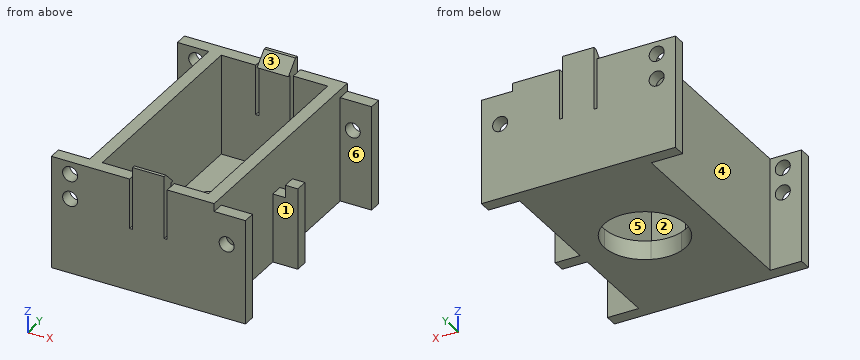
```python
from build123d import *

# Parameters (mm, degrees)
F1_DEPTH  = 2
F2_DEPTH  = 18
F3_DEPTH  = 3
F4_W      = 2
F4_H      = 5
F4_H_2    = 13
F5_DEPTH  = 5
F6_W      = 2
F6_H      = 16.7173967883
F7_DEPTH  = 5
F8_R      = 1.2
F9_DEPTH  = 40
F12_DEPTH = 1
F13_W     = 5
F13_H     = 2
F13_H_2   = 0.5
F14_DEPTH = 2
F15_SIZE  = 1.99999
F13_W_2   = 0.5
F16_DEPTH = 8


# Not quite as in the source:
# - a fillet or chamfer is up to 0.001 mm smaller than in the source, because OpenCascade refuses the exact size


with BuildPart() as f1:
    # F0 (on Top) → F1 (new body)
    with BuildSketch(Plane.XY):
        Polygon((-5.1606558692, 9.7513413054), (-11.6606558692, 9.7513413054), (-11.6606558692, -27.7486586946), (-5.1606558692, -27.7486586946), (2.8393441308, -27.7486586946), (9.3393441308, -27.7486586946), (9.3393441308, 9.7513413054), (2.8393441308, 9.7513413054), align=None)
        Polygon((-9.6606558692, -1.2486586946), (-9.6606558692, 7.7513413054), (7.3393441308, 7.7513413054), (7.3393441308, -1.2486586946), (7.3393441308, -16.7486586946), (7.3393441308, -25.7486586946), (-9.6606558692, -25.7486586946), (-9.6606558692, -16.7486586946), align=None, mode=Mode.SUBTRACT)
        with BuildLine():
            Line((3.3125979801, -16.7486586946), (-5.6339097184, -16.7486586946))
            ThreePointArc((-5.6339097184, -16.7486586946), (-2.8409986659, -25.1856853401), (4.3393441308, -19.9486586946))
            ThreePointArc((4.3393441308, -19.9486586946), (4.0763707763, -18.2683158979), (3.3125979801, -16.7486586946))
        make_face()
        with BuildLine():
            ThreePointArc((4.3393441308, 1.9513413054), (-2.8409986659, 7.1883679509), (-5.6339097184, -1.2486586946))
            Line((-5.6339097184, -1.2486586946), (3.3125979801, -1.2486586946))
            ThreePointArc((3.3125979801, -1.2486586946), (4.0763707763, 0.2709985087), (4.3393441308, 1.9513413054))
        make_face()
        with BuildLine():
            Line((7.3393441308, 7.7513413054), (-9.6606558692, 7.7513413054))
            Line((-9.6606558692, 7.7513413054), (-9.6606558692, -1.2486586946))
            Line((-9.6606558692, -1.2486586946), (-5.6339097184, -1.2486586946))
            ThreePointArc((-5.6339097184, -1.2486586946), (-2.8409986659, 7.1883679509), (4.3393441308, 1.9513413054))
            ThreePointArc((4.3393441308, 1.9513413054), (4.0763707763, 0.2709985087), (3.3125979801, -1.2486586946))
            Line((3.3125979801, -1.2486586946), (7.3393441308, -1.2486586946))
            Line((7.3393441308, -1.2486586946), (7.3393441308, 7.7513413054))
        make_face()
        with BuildLine():
            Line((-5.6339097184, -16.7486586946), (-9.6606558692, -16.7486586946))
            Line((-9.6606558692, -16.7486586946), (-9.6606558692, -25.7486586946))
            Line((-9.6606558692, -25.7486586946), (7.3393441308, -25.7486586946))
            Line((7.3393441308, -25.7486586946), (7.3393441308, -16.7486586946))
            Line((7.3393441308, -16.7486586946), (3.3125979801, -16.7486586946))
            ThreePointArc((3.3125979801, -16.7486586946), (4.0763707763, -18.2683158979), (4.3393441308, -19.9486586946))
            ThreePointArc((4.3393441308, -19.9486586946), (-2.8409986659, -25.1856853401), (-5.6339097184, -16.7486586946))
        make_face()
        with BuildLine():
            Line((7.3393441308, -16.7486586946), (7.3393441308, -1.2486586946))
            Line((7.3393441308, -1.2486586946), (3.3125979801, -1.2486586946))
            ThreePointArc((3.3125979801, -1.2486586946), (2.6358545698, -2.028169781), (1.8253711817, -2.667494311))
            ThreePointArc((1.8253711817, -2.667494311), (4.751289215, -5.2504717566), (5.8393441308, -8.9986586946))
            ThreePointArc((5.8393441308, -8.9986586946), (4.751289215, -12.7468456326), (1.8253711817, -15.3298230782))
            ThreePointArc((1.8253711817, -15.3298230782), (2.6358545698, -15.9691476082), (3.3125979801, -16.7486586946))
            Line((3.3125979801, -16.7486586946), (7.3393441308, -16.7486586946))
        make_face()
        with BuildLine():
            Line((-5.6339097184, -1.2486586946), (-9.6606558692, -1.2486586946))
            Line((-9.6606558692, -1.2486586946), (-9.6606558692, -16.7486586946))
            Line((-9.6606558692, -16.7486586946), (-5.6339097184, -16.7486586946))
            ThreePointArc((-5.6339097184, -16.7486586946), (-4.9571663082, -15.9691476082), (-4.14668292, -15.3298230782))
            ThreePointArc((-4.14668292, -15.3298230782), (-8.1606558692, -8.9986586946), (-4.14668292, -2.667494311))
            ThreePointArc((-4.14668292, -2.667494311), (-4.9571663082, -2.028169781), (-5.6339097184, -1.2486586946))
        make_face()
        with BuildLine():
            Line((3.3125979801, -1.2486586946), (-5.6339097184, -1.2486586946))
            ThreePointArc((-5.6339097184, -1.2486586946), (-4.9571663082, -2.028169781), (-4.14668292, -2.667494311))
            ThreePointArc((-4.14668292, -2.667494311), (-1.1606558692, -1.9986586946), (1.8253711817, -2.667494311))
            ThreePointArc((1.8253711817, -2.667494311), (2.6358545698, -2.028169781), (3.3125979801, -1.2486586946))
        make_face()
        with BuildLine():
            ThreePointArc((-4.14668292, -15.3298230782), (-4.9571663082, -15.9691476082), (-5.6339097184, -16.7486586946))
            Line((-5.6339097184, -16.7486586946), (3.3125979801, -16.7486586946))
            ThreePointArc((3.3125979801, -16.7486586946), (2.6358545698, -15.9691476082), (1.8253711817, -15.3298230782))
            ThreePointArc((1.8253711817, -15.3298230782), (-1.1606558692, -15.9986586946), (-4.14668292, -15.3298230782))
        make_face()
    extrude(amount=F1_DEPTH)

    # F0 (on Top) → F2 (join)
    with BuildSketch(Plane.XY):
        Polygon((-5.1606558692, 9.7513413054), (-11.6606558692, 9.7513413054), (-11.6606558692, -27.7486586946), (-5.1606558692, -27.7486586946), (2.8393441308, -27.7486586946), (9.3393441308, -27.7486586946), (9.3393441308, 9.7513413054), (2.8393441308, 9.7513413054), align=None)
        Polygon((-9.6606558692, -1.2486586946), (-9.6606558692, 7.7513413054), (7.3393441308, 7.7513413054), (7.3393441308, -1.2486586946), (7.3393441308, -16.7486586946), (7.3393441308, -25.7486586946), (-9.6606558692, -25.7486586946), (-9.6606558692, -16.7486586946), align=None, mode=Mode.SUBTRACT)
    extrude(amount=F2_DEPTH)

    # F0 (on Top) → F3 (join)
    with BuildSketch(Plane.XY):
        with BuildLine():
            ThreePointArc((-3.604859431, -2.9757134891), (-3.8801412786, -2.8292861752), (-4.14668292, -2.667494311))
            ThreePointArc((-4.14668292, -2.667494311), (-8.1606558692, -8.9986586946), (-4.14668292, -15.3298230782))
            ThreePointArc((-4.14668292, -15.3298230782), (-3.8801412786, -15.1680312141), (-3.604859431, -15.0216039001))
            ThreePointArc((-3.604859431, -15.0216039001), (-7.6606558692, -8.9986586946), (-3.604859431, -2.9757134891))
        make_face()
        with BuildLine():
            ThreePointArc((1.8253711817, -2.667494311), (-1.1606558692, -1.9986586946), (-4.14668292, -2.667494311))
            ThreePointArc((-4.14668292, -2.667494311), (-3.8801412786, -2.8292861752), (-3.604859431, -2.9757134891))
            ThreePointArc((-3.604859431, -2.9757134891), (-1.1606558692, -2.4986586946), (1.2835476927, -2.9757134891))
            ThreePointArc((1.2835476927, -2.9757134891), (1.5588295403, -2.8292861752), (1.8253711817, -2.667494311))
        make_face()
        with BuildLine():
            ThreePointArc((5.8393441308, -8.9986586946), (4.751289215, -5.2504717566), (1.8253711817, -2.667494311))
            ThreePointArc((1.8253711817, -2.667494311), (1.5588295403, -2.8292861752), (1.2835476927, -2.9757134891))
            ThreePointArc((1.2835476927, -2.9757134891), (4.2308802362, -5.3680473929), (5.3393441308, -8.9986586946))
            ThreePointArc((5.3393441308, -8.9986586946), (4.2308802362, -12.6292699963), (1.2835476927, -15.0216039001))
            ThreePointArc((1.2835476927, -15.0216039001), (1.5588295403, -15.1680312141), (1.8253711817, -15.3298230782))
            ThreePointArc((1.8253711817, -15.3298230782), (4.751289215, -12.7468456326), (5.8393441308, -8.9986586946))
        make_face()
        with BuildLine():
            ThreePointArc((-3.604859431, -15.0216039001), (-3.8801412786, -15.1680312141), (-4.14668292, -15.3298230782))
            ThreePointArc((-4.14668292, -15.3298230782), (-1.1606558692, -15.9986586946), (1.8253711817, -15.3298230782))
            ThreePointArc((1.8253711817, -15.3298230782), (1.5588295403, -15.1680312141), (1.2835476927, -15.0216039001))
            ThreePointArc((1.2835476927, -15.0216039001), (-1.1606558692, -15.4986586946), (-3.604859431, -15.0216039001))
        make_face()
    extrude(amount=F3_DEPTH)

    # F4 (on face) → F5 (join)
    with BuildSketch(Plane(origin=(-11.6606558692, 0, 0), x_dir=(0, -1, 0), z_dir=(-1, 0, 0))):
        with Locations((-8.7513413054, 2.5)):
            Rectangle(F4_W, F4_H)
        with Locations((-8.7513413054, 11.5)):
            Rectangle(F4_W, F4_H_2)
        with Locations((26.7486586946, 2.5)):
            Rectangle(F4_W, F4_H)
        with Locations((26.7486586946, 11.5)):
            Rectangle(F4_W, F4_H_2)
    extrude(amount=F5_DEPTH)

    # F6 (on face) → F7 (join)
    with BuildSketch(Plane.YZ.offset(9.3393441308)):
        with Locations((-26.7486586946, 8.3586983941)):
            Rectangle(F6_W, F6_H)
        with Locations((8.7513413054, 8.3586983941)):
            Rectangle(F6_W, F6_H)
    extrude(amount=F7_DEPTH)

    # F8 (on face) → F9 (cut)
    with BuildSketch(Plane.XZ.offset(27.7486586946)):
        with Locations((-13.6606558692, 12)):
            Circle(F8_R)
        with Locations((11.3393441308, 12)):
            Circle(F8_R)
        with Locations((-13.6606558692, 16)):
            Circle(F8_R)
    extrude(amount=-F9_DEPTH, mode=Mode.SUBTRACT)

    # F11 (on offset) → F12 (join, symmetric)
    with BuildSketch(Plane(origin=(0, -10.2486586946, 0), x_dir=(-1, 0, 0), z_dir=(0, 1, 0))):
        Polygon((-13.3393441308, 13), (-13.3393441308, 0), (-9.3393441308, 0), (-9.3393441308, 11), (-11.3393441308, 11), (-11.3393441308, 13), align=None)
    extrude(amount=F12_DEPTH, both=True)

    # F13 (on face) → F14 (join)
    with BuildSketch(Plane.XY.offset(18)):
        with Locations((-1.1606558692, -26.7486586946)):
            Rectangle(F13_W, F13_H)
        with Locations((-1.1606558692, -25.4986586946)):
            Rectangle(F13_W, F13_H_2)
        with Locations((-1.1606558692, 8.7513413054)):
            Rectangle(F13_W, F13_H)
        with Locations((-1.1606558692, 7.5013413054)):
            Rectangle(F13_W, F13_H_2)
    extrude(amount=F14_DEPTH)

    # F15 (size 2 in the source; OpenCascade refuses exactly that, so slightly less here)
    f15_edges = [f1.edges().sort_by_distance(p)[0] for p in [
        (-1.160656, -25.248659, 20),
        (-1.160656, 7.251341, 20),
    ]]
    chamfer(f15_edges, length=F15_SIZE)

    # F13 (on face) → F16 (cut)
    with BuildSketch(Plane.XY.offset(18)):
        with Locations((-3.9106558692, -26.7486586946)):
            Rectangle(F13_W_2, F13_H)
        with Locations((1.5893441308, -26.7486586946)):
            Rectangle(F13_W_2, F13_H)
        with Locations((1.5893441308, 8.7513413054)):
            Rectangle(F13_W_2, F13_H)
        with Locations((-3.9106558692, 8.7513413054)):
            Rectangle(F13_W_2, F13_H)
    extrude(amount=-F16_DEPTH, mode=Mode.SUBTRACT)


solid = f1.part
```
Work out the finished part from the listing and answer in its coordinate system (mm). Face numbers are marked on the shaded views. A direction names the side the tool comes from. Coordinates: 2 decimals unless noted, no trailing zeros. Write each loop counter-clockwise with the first axis right and the second up, starting at its lowest first coordinate (ties: lowest second). Pieces come first, ordered by that corner, then holes.
Q1. A cutting plane is placed at A-A, the plane z = 4. Give the vertices of the cut face in (x, y).
Q2. A cutting plane is placed at B-B, the plane x = -13. Give the vertices of the cut face in (y, z).
Q3. Each of these flat-tipped pins is pushed along its axis until it touches: pin 1 Ø2 at (x, y) = (10.5, -14.5) entering from +Z; pin 2 Ø4 at (x, y) = (7, -10.5) entering from +Z; pin 3 Ø1.9 at (x, z) = (11.34, 12) entering from +Y; pin 4 Ø13.5 at (x, y) = (-2.5, -1.5) entering from +Z. Where does it stop, or does it pass through?
Q4. A cutting plane is placed at C-C, the plane x = 12. Give the vertices of the cut face in (y, z).
Q5. Which of the six approach directions +Z, -Z, +X, -X, +Y, -Y give full straight-line access (tool end or side, diameter ignored) to the marked faces 1, 2 and 3?
Q6. Determine the mould class of the marked faces 4, 5 and 6 for opening direction X: released by +X, released by -X, zero draft, split by the parting line, or undercut.
Q7. Find the intervals of material crossed by line 1 (Y direction, x = 11, z = 9.75); line 2 (Z direction, x = 12, y = -26); line 3 (X direction, y = -9, z = 15), in increasing order.
Q8. A cutting plane is placed at D-D, the plane y = -23. Give the vertices of the cut face in (x, z), then the cut area to 3 significant figures.
Findings below:
1. outline: (-16.66, -27.75) - (14.34, -27.75) - (14.34, -25.75) - (9.34, -25.75) - (9.34, -11.25) - (13.34, -11.25) - (13.34, -9.25) - (9.34, -9.25) - (9.34, 7.75) - (14.34, 7.75) - (14.34, 9.75) - (-16.66, 9.75) - (-16.66, 7.75) - (-11.66, 7.75) - (-11.66, -25.75) - (-16.66, -25.75) - close; hole (-9.66, -25.75) - (7.34, -25.75) - (7.34, 7.75) - (-9.66, 7.75) - close
2. outline: (-27.75, 0) - (-25.75, 0) - (-25.75, 11) - (-27.75, 11) - close; (-27.75, 13) - (-25.75, 13) - (-25.75, 15) - (-27.75, 15) - close; (-27.75, 17) - (-25.75, 17) - (-25.75, 18) - (-27.75, 18) - close; (7.75, 0) - (9.75, 0) - (9.75, 11) - (7.75, 11) - close; (7.75, 13) - (9.75, 13) - (9.75, 15) - (7.75, 15) - close; (7.75, 17) - (9.75, 17) - (9.75, 18) - (7.75, 18) - close
3. pin 1: passes through
3. pin 2: stops at z = 18
3. pin 3: stops at y = -9.25
3. pin 4: stops at z = 3
4. outline: (-27.75, 0) - (-25.75, 0) - (-25.75, 11) - (-27.75, 11) - close; (-27.75, 13) - (-25.75, 13) - (-25.75, 16.72) - (-27.75, 16.72) - close; (-11.25, 0) - (-9.25, 0) - (-9.25, 13) - (-11.25, 13) - close; (7.75, 0) - (9.75, 0) - (9.75, 11) - (7.75, 11) - close; (7.75, 13) - (9.75, 13) - (9.75, 16.72) - (7.75, 16.72) - close
5. face 1: +Z, -Z, +X
5. face 2: none
5. face 3: +Z, +X, -X
6. face 4: released by -X
6. face 5: undercut
6. face 6: zero draft
7. line 1: y = -27.75 to -25.75, -11.25 to -9.25, 7.75 to 9.75
7. line 2: z = 0 to 11, 13 to 16.72
7. line 3: x = -11.66 to -9.66, 7.34 to 9.34
8. outline: (-11.66, 0) - (9.34, 0) - (9.34, 18) - (7.34, 18) - (7.34, 2) - (-9.66, 2) - (-9.66, 18) - (-11.66, 18) - close
8. area: 106 mm2
